For this review, take the finished solid that the model builds, in its own axes (mm). A direction names the side the tool comes from. Give positions to 0.01 mm unless a question says otherwise; leave off trailing zeros. Write each loop counter-clockwise with the first axis right and the second up, starting at its lowest first coordinate (ties: lowest second). Pieces come first, ordered by that corner, then holes. Notation, with made-up numbers: M 32,82.25 L 80,82.25 A22 ccw 80,107.25 Z; hole C 33,70.25 d1. An arc over 180 degrees is marked long. Write item = value, one per line.
```python
from build123d import *

# Parameters (mm, degrees)
SKETCH1_W           = 80
SKETCH1_H           = 48
SKETCH1_W_2         = 76
SKETCH1_H_2         = 44
BOSS_EXTRUDE1_DEPTH = 6
SKETCH2_W           = 80
SKETCH2_H           = 48
SKETCH2_W_2         = 74
SKETCH2_H_2         = 42
BOSS_EXTRUDE2_DEPTH = 1
FILLET1_R           = 3
SKETCH3_W           = 5
SKETCH3_H           = 1.5
SKETCH3_W_2         = 1.5
SKETCH3_H_2         = 3
BOSS_EXTRUDE3_DEPTH = 1.5
CHAMFER2_SIZE       = 1.5


with BuildPart() as part:
    # Sketch1 → Boss-Extrude1 (new body)
    with BuildSketch(Plane(origin=(0, 0, 0), x_dir=(1, 0, 0), z_dir=(0, 1, 0))):
        Rectangle(SKETCH1_W, SKETCH1_H)
        Rectangle(SKETCH1_W_2, SKETCH1_H_2, mode=Mode.SUBTRACT)
    extrude(amount=BOSS_EXTRUDE1_DEPTH)

    # Sketch2 → Boss-Extrude2 (add)
    with BuildSketch(Plane(origin=(0, 6, 0), x_dir=(1, 0, 0), z_dir=(0, 1, 0))):
        Rectangle(SKETCH2_W, SKETCH2_H)
        Rectangle(SKETCH2_W_2, SKETCH2_H_2, mode=Mode.SUBTRACT)
    extrude(amount=BOSS_EXTRUDE2_DEPTH)

    # Fillet1
    fillet1_edges = [part.edges().sort_by_distance(p)[0] for p in [
        (40, 3.5, -24),
        (40, 3.5, 24),
        (-40, 3.5, 24),
        (-40, 3.5, -24),
    ]]
    fillet(fillet1_edges, radius=FILLET1_R)

    # Sketch3 → Boss-Extrude3 (add)
    with BuildSketch(Plane.XZ):
        with Locations((-23.5, 21.25)):
            Rectangle(SKETCH3_W, SKETCH3_H)
        with Locations((-37.25, 12.5)):
            Rectangle(SKETCH3_W_2, SKETCH3_H_2)
        with Locations((23.5, 21.25)):
            Rectangle(SKETCH3_W, SKETCH3_H)
        with Locations((-37.25, -12.5)):
            Rectangle(SKETCH3_W_2, SKETCH3_H_2)
    extrude(amount=-BOSS_EXTRUDE3_DEPTH)

    # Chamfer2
    chamfer2_edges = [part.edges().sort_by_distance(p)[0] for p in [
        (23.5, 0, 20.5),
        (-23.5, 0, 20.5),
        (-36.5, 0, -12.5),
        (-36.5, 0, 12.5),
    ]]
    chamfer(chamfer2_edges, length=CHAMFER2_SIZE - 0.0001)  # a hair under: the kernel refuses the full size


solid = part.part
```
1. The part is to be moulded in two halves that separate along X. For faces 4 (the face through (-3.1, 7, 21.2)), 5 (the face through (-39.14, 3.45, -23.1)), 6 (the face through (23, 1.5, 21)), say which applies: +X half, -X half, draft (parallel to the pull), parting line (faces both ways), or undercut.
Responses:
face_4 = draft
face_5 = -X half
face_6 = undercut
2. We need section B-B, the plane x = -4. Write out the cut boundary in (y, z), then the cut area to 3 significant figures.
Responses:
outline = M 0,-24 L 7,-24 L 7,-21 L 6,-21 L 6,-22 L 0,-22 Z; M 0,22 L 6,22 L 6,21 L 7,21 L 7,24 L 0,24 Z
area = 30.0 mm2
3. We need section C-C, the plane y = 5.25. Write out the cut boundary in (x, z).
Responses:
outline = M -40,-21 A3 ccw -37,-24 L 37,-24 A3 ccw 40,-21 L 40,21 A3 ccw 37,24 L -37,24 A3 ccw -40,21 Z; hole M -38,-22 L 38,-22 L 38,22 L -38,22 Z
4. For line 1 along X through (y, z) = (5.5, 17); line 2 along Z through (x, y) = (-18, 4.5); line 3 along X through (y, z) = (6.25, 1.5), list the stretches that pass through material, from the lowest coordinate up. Write a range as from..to.
Responses:
line_1 = -40..-38, 38..40
line_2 = -24..-22, 22..24
line_3 = -40..-37, 37..40
5. Machinability: for faces 1 (the face through (-37, 1.5, -12)), 2 (the face through (23, 1, 21)), 3 (the face through (-39.14, 3.55, 23.1)), which of the approach directions +Z, -Z, +X, -X, +Y, -Y give a long, thin tool a straight path to every point of the face, cutting with its end or side? Answer none if there is none.
Responses:
face_1 = none
face_2 = -Y
face_3 = +Z, -X, +Y, -Y
6. We need section D-D, the plane z = 5.5. Write out the cut boundary in (x, y), then the cut area to 3 significant figures.
Responses:
outline = M -40,0 L -38,0 L -38,6 L -37,6 L -37,7 L -40,7 Z; M 37,6 L 38,6 L 38,0 L 40,0 L 40,7 L 37,7 Z
area = 30.0 mm2
